Geometry: final body of the model. Coordinates: model frame, mm. Face numbers are marked on the shaded views. A direction names the side the tool comes from. Give positions to 0.01 mm unless a question says otherwise; leave off trailing zeros. Write each loop counter-clockwise with the first axis right and the second up, starting at its lowest first coordinate (ties: lowest second). Pieces come first, ordered by that corner, then holes.
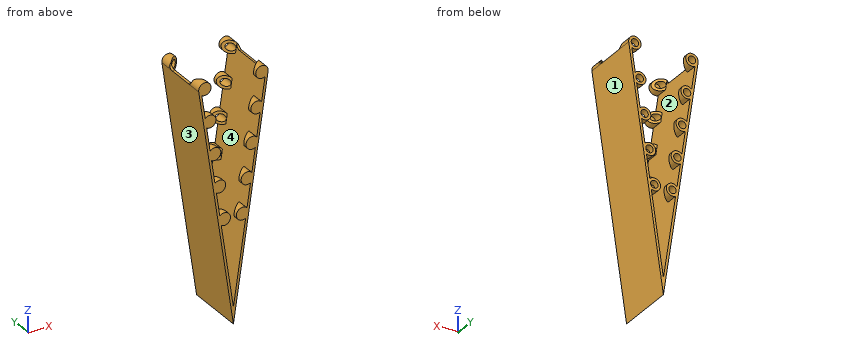
from build123d import *

# Parameters (mm, degrees)
BOSS_EXTRUDE1_DEPTH            = 25
SKETCH2_R                      = 2.6
SKETCH2_R_2                    = 1.55
BOSS_EXTRUDE3_DEPTH            = 5
CUT_EXTRUDE1_REACH             = 107.119
CUT_EXTRUDE1_DIRECTION_2_DEPTH = 106.119492302
CUT_EXTRUDE2_REACH             = 107.119
CUT_EXTRUDE2_DIRECTION_2_DEPTH = 106.119492302
FILLET1_R                      = 2
SKETCH6_R                      = 1.55
BOSS_EXTRUDE4_DEPTH            = 1


with BuildPart() as part:
    # Sketch1 → Boss-Extrude1 (new body)
    with BuildSketch(Plane(origin=(0, 0, 0), x_dir=(1, 0, 0), z_dir=(0, 1, 0))):
        Polygon((-13.5, 0), (0, 92.188031325), (13.5, 0), (14.489447114, 0.144894471), (0, 99.089605913), (-14.489447114, 0.144894471), align=None)
    extrude(amount=BOSS_EXTRUDE1_DEPTH)

    # Sketch2 → Boss-Extrude3 (add)
    # profile 1 of 10: a face of its own
    with BuildSketch(Plane(origin=(0, 0, 0), x_dir=(1, 0, 0), z_dir=(0, 1, 0))):
        with Locations((11.916884617, -0.231831154)):
            Circle(SKETCH2_R)
        with Locations(Location((11.916884617, -0.231831154, 0), (0, 0, 270))):
            Circle(SKETCH2_R_2, mode=Mode.SUBTRACT)
    # profile 2 of 10: a face of its own
    with BuildSketch(Plane(origin=(0, 0, 0), x_dir=(1, 0, 0), z_dir=(0, 1, 0))):
        with Locations((9.888362021, 13.620428448)):
            Circle(SKETCH2_R)
        with Locations(Location((9.888362021, 13.620428448, 0), (0, 0, 270))):
            Circle(SKETCH2_R_2, mode=Mode.SUBTRACT)
    # profile 3 of 10: a face of its own
    with BuildSketch(Plane(origin=(0, 0, 0), x_dir=(1, 0, 0), z_dir=(0, 1, 0))):
        with Locations((7.859839425, 27.47268805)):
            Circle(SKETCH2_R)
        with Locations(Location((7.859839425, 27.47268805, 0), (0, 0, 270))):
            Circle(SKETCH2_R_2, mode=Mode.SUBTRACT)
    # profile 4 of 10: a face of its own
    with BuildSketch(Plane(origin=(0, 0, 0), x_dir=(1, 0, 0), z_dir=(0, 1, 0))):
        with Locations((5.831316829, 41.324947652)):
            Circle(SKETCH2_R)
        with Locations(Location((5.831316829, 41.324947652, 0), (0, 0, 270))):
            Circle(SKETCH2_R_2, mode=Mode.SUBTRACT)
    # profile 5 of 10: a face of its own
    with BuildSketch(Plane(origin=(0, 0, 0), x_dir=(1, 0, 0), z_dir=(0, 1, 0))):
        with Locations((3.802794233, 55.177207254)):
            Circle(SKETCH2_R)
        with Locations(Location((3.802794233, 55.177207254, 0), (0, 0, 270))):
            Circle(SKETCH2_R_2, mode=Mode.SUBTRACT)
    # profile 6 of 10: a face of its own
    with BuildSketch(Plane(origin=(0, 0, 0), x_dir=(1, 0, 0), z_dir=(0, 1, 0))):
        with Locations((-11.916884617, -0.231831154)):
            Circle(SKETCH2_R)
        with Locations(Location((-11.916884617, -0.231831154, 0), (0, 0, 90))):
            Circle(SKETCH2_R_2, mode=Mode.SUBTRACT)
    # profile 7 of 10: a face of its own
    with BuildSketch(Plane(origin=(0, 0, 0), x_dir=(1, 0, 0), z_dir=(0, 1, 0))):
        with Locations((-9.888362021, 13.620428448)):
            Circle(SKETCH2_R)
        with Locations(Location((-9.888362021, 13.620428448, 0), (0, 0, 90))):
            Circle(SKETCH2_R_2, mode=Mode.SUBTRACT)
    # profile 8 of 10: a face of its own
    with BuildSketch(Plane(origin=(0, 0, 0), x_dir=(1, 0, 0), z_dir=(0, 1, 0))):
        with Locations((-7.859839425, 27.47268805)):
            Circle(SKETCH2_R)
        with Locations(Location((-7.859839425, 27.47268805, 0), (0, 0, 90))):
            Circle(SKETCH2_R_2, mode=Mode.SUBTRACT)
    # profile 9 of 10: a face of its own
    with BuildSketch(Plane(origin=(0, 0, 0), x_dir=(1, 0, 0), z_dir=(0, 1, 0))):
        with Locations((-5.831316829, 41.324947652)):
            Circle(SKETCH2_R)
        with Locations(Location((-5.831316829, 41.324947652, 0), (0, 0, 90))):
            Circle(SKETCH2_R_2, mode=Mode.SUBTRACT)
    # profile 10 of 10: a face of its own
    with BuildSketch(Plane(origin=(0, 0, 0), x_dir=(1, 0, 0), z_dir=(0, 1, 0))):
        with Locations((-3.802794233, 55.177207254)):
            Circle(SKETCH2_R)
        with Locations(Location((-3.802794233, 55.177207254, 0), (0, 0, 90))):
            Circle(SKETCH2_R_2, mode=Mode.SUBTRACT)
    boss_extrude3 = extrude(amount=BOSS_EXTRUDE3_DEPTH)

    # Cut-Extrude1: up to this face of the body (flat: up to its plane)
    cut_extrude1_end = Plane(part.part.faces().sort_by_distance((-6.65824674, 12.912249129, -46.7205751))[0])
    # Sketch4 → Cut-Extrude1 (cut, up to the picked face)
    with BuildSketch(Plane(origin=(0.283424505, 0, 1.935433121), x_dir=(0.9894471144188783, 0, -0.14489447114419254), z_dir=(0.14489447114419252, 0, 0.9894471144188782)), mode=Mode.PRIVATE) as cut_extrude1_sk1:
        Polygon((13.357536045, 5), (9.157536045, 5), (9.157536045, 1.475781549), align=None)
    cut_extrude1_tool1 = split(extrude(cut_extrude1_sk1.sketch, amount=-CUT_EXTRUDE1_REACH, mode=Mode.PRIVATE), bisect_by=cut_extrude1_end, keep=Keep.BOTH, mode=Mode.PRIVATE)
    cut_extrude1 = cut_extrude1_tool1.solids().sort_by(Axis((10.729548, 3.825261, 0.405705), (-0.14489447114419252, 0, -0.9894471144188782)))[0]
    add(cut_extrude1, mode=Mode.SUBTRACT)

    # Sketch4 → Cut-Extrude1 direction 2 (cut)
    with BuildSketch(Plane(origin=(0.283424505, 0, 1.935433121), x_dir=(0.9894471144188783, 0, -0.14489447114419254), z_dir=(0.14489447114419252, 0, 0.9894471144188782))):
        Polygon((13.357536045, 5), (9.157536045, 5), (9.157536045, 1.475781549), align=None)
    cut_extrude1_direction_2 = extrude(amount=CUT_EXTRUDE1_DIRECTION_2_DEPTH, mode=Mode.SUBTRACT)

    # Cut-Extrude2: up to this face of the body (flat: up to its plane)
    cut_extrude2_end = Plane(part.part.faces().sort_by_distance((6.65824674, 12.912249129, -46.7205751))[0])
    # Sketch5 → Cut-Extrude2 (cut, up to the picked face)
    with BuildSketch(Plane(origin=(-0.283424505, 0, 1.935433121), x_dir=(0.9894471144188784, 0, 0.14489447114419146), z_dir=(-0.14489447114419146, 0, 0.9894471144188784)), mode=Mode.PRIVATE) as cut_extrude2_sk1:
        Polygon((-9.157536045, 5), (-9.157536045, 1.475781549), (-13.357536045, 5), align=None)
    cut_extrude2_tool1 = split(extrude(cut_extrude2_sk1.sketch, amount=-CUT_EXTRUDE2_REACH, mode=Mode.PRIVATE), bisect_by=cut_extrude2_end, keep=Keep.BOTH, mode=Mode.PRIVATE)
    cut_extrude2 = cut_extrude2_tool1.solids().sort_by(Axis((-10.729548, 3.825261, 0.405705), (0.14489447114419146, 0, -0.9894471144188784)))[0]
    add(cut_extrude2, mode=Mode.SUBTRACT)

    # Sketch5 → Cut-Extrude2 direction 2 (cut)
    with BuildSketch(Plane(origin=(-0.283424505, 0, 1.935433121), x_dir=(0.9894471144188784, 0, 0.14489447114419146), z_dir=(-0.14489447114419146, 0, 0.9894471144188784))):
        Polygon((-9.157536045, 5), (-9.157536045, 1.475781549), (-13.357536045, 5), align=None)
    cut_extrude2_direction_2 = extrude(amount=CUT_EXTRUDE2_DIRECTION_2_DEPTH, mode=Mode.SUBTRACT)

    # Mirror2: Boss-Extrude3, Cut-Extrude1, Cut-Extrude1 direction 2, Cut-Extrude2, Cut-Extrude2 direction 2 across plane
    add(boss_extrude3.mirror(Plane.ZX.offset(12.5)))
    add(cut_extrude1.mirror(Plane.ZX.offset(12.5)), mode=Mode.SUBTRACT)
    add(cut_extrude1_direction_2.mirror(Plane.ZX.offset(12.5)), mode=Mode.SUBTRACT)
    add(cut_extrude2.mirror(Plane.ZX.offset(12.5)), mode=Mode.SUBTRACT)
    add(cut_extrude2_direction_2.mirror(Plane.ZX.offset(12.5)), mode=Mode.SUBTRACT)

    # Fillet1
    # the kernel refuses this fillet: 2 mm, written as the material it adds along each edge
    with BuildSketch(Plane(origin=(13.5, 5, 0), x_dir=(0, 1, 0), z_dir=(0.9894471144188783, 0, -0.1448944711441925))) as fillet1_piece_1_section:
        with BuildLine():
            CenterArc((FILLET1_R, FILLET1_R), FILLET1_R, 180, 90)
            Line((0, FILLET1_R), (0, 0))
            Line((0, 0), (FILLET1_R, 0))
        make_face()
    fillet1_piece_1 = extrude(amount=6, mode=Mode.PRIVATE)
    fillet1_piece_1 = fillet1_piece_1 & Plane(origin=(11.916884617, 5, 0.231831154), x_dir=(1, 0, 0), z_dir=(0, -1, 0)) * Cylinder(2.6, 20, mode=Mode.PRIVATE)
    add(fillet1_piece_1)
    with BuildSketch(Plane(origin=(13.5, 20, 0), x_dir=(0, -1, 0), z_dir=(0.9894471144188783, 0, -0.1448944711441925))) as fillet1_piece_2_section:
        with BuildLine():
            CenterArc((FILLET1_R, -FILLET1_R), FILLET1_R, 90, 90)
            Line((0, -FILLET1_R), (0, 0))
            Line((0, 0), (FILLET1_R, 0))
        make_face()
    fillet1_piece_2 = extrude(amount=6, mode=Mode.PRIVATE)
    fillet1_piece_2 = fillet1_piece_2 & Plane(origin=(11.916884617, 20, 0.231831154), x_dir=(1, 0, 0), z_dir=(0, 1, 0)) * Cylinder(2.6, 20, mode=Mode.PRIVATE)
    add(fillet1_piece_2)
    with BuildSketch(Plane(origin=(-19.436682687, 20, -0.869366827), x_dir=(0, -1, 0), z_dir=(0.9894471144188784, 0, 0.1448944711441914))) as fillet1_piece_3_section:
        with BuildLine():
            CenterArc((FILLET1_R, -FILLET1_R), FILLET1_R, 90, 90)
            Line((0, -FILLET1_R), (0, 0))
            Line((0, 0), (FILLET1_R, 0))
        make_face()
    fillet1_piece_3 = extrude(amount=6, mode=Mode.PRIVATE)
    fillet1_piece_3 = fillet1_piece_3 & Plane(origin=(-11.916884617, 20, 0.231831154), x_dir=(1, 0, 0), z_dir=(0, 1, 0)) * Cylinder(2.6, 21, mode=Mode.PRIVATE)
    add(fillet1_piece_3)
    with BuildSketch(Plane(origin=(-19.436682687, 5, -0.869366827), x_dir=(-0.1448944711441914, 0, 0.9894471144188784), z_dir=(0.9894471144188784, 0, 0.1448944711441914))) as fillet1_piece_4_section:
        with BuildLine():
            CenterArc((FILLET1_R, -FILLET1_R), FILLET1_R, 90, 90)
            Line((0, -FILLET1_R), (0, 0))
            Line((0, 0), (FILLET1_R, 0))
        make_face()
    fillet1_piece_4 = extrude(amount=6, mode=Mode.PRIVATE)
    fillet1_piece_4 = fillet1_piece_4 & Plane(origin=(-11.916884617, 5, 0.231831154), x_dir=(1, 0, 0), z_dir=(0, -1, 0)) * Cylinder(2.6, 21, mode=Mode.PRIVATE)
    add(fillet1_piece_4)

    # Sketch6 → Boss-Extrude4 (add)
    with BuildSketch(Plane.XZ):
        with Locations(Location((3.802794233, -55.177207254, 0), (0, 0, 270))):
            Circle(SKETCH6_R)
        with Locations(Location((-3.802794233, -55.177207254, 0), (0, 0, 270))):
            Circle(SKETCH6_R)
        with Locations(Location((-5.831316829, -41.324947652, 0), (0, 0, 270))):
            Circle(SKETCH6_R)
        with Locations(Location((5.831316829, -41.324947652, 0), (0, 0, 270))):
            Circle(SKETCH6_R)
        with Locations(Location((7.859839425, -27.47268805, 0), (0, 0, 270))):
            Circle(SKETCH6_R)
        with Locations(Location((-7.859839425, -27.47268805, 0), (0, 0, 270))):
            Circle(SKETCH6_R)
        with Locations(Location((-9.888362021, -13.620428448, 0), (0, 0, 270))):
            Circle(SKETCH6_R)
        with Locations(Location((9.888362021, -13.620428448, 0), (0, 0, 270))):
            Circle(SKETCH6_R)
        with Locations(Location((11.916884617, 0.231831154, 0), (0, 0, 270))):
            Circle(SKETCH6_R)
        with Locations(Location((-11.916884617, 0.231831154, 0), (0, 0, 270))):
            Circle(SKETCH6_R)
    extrude(amount=-BOSS_EXTRUDE4_DEPTH)


solid = part.part
Q1. Access query for the marked faces 3 and 4. Directions: +Z, -Z, +X, -X, +Y, -Y. A direction counts if a zero-diameter tool reaches every point of the face in a straight line with its end or side. Return the directions, or none.
Filled sheet:
face 3: -Z, -X, +Y, -Y
face 4: none
Q2. Section B-B on y = 15.75. Output: boundary loops of the cut face in (x, z), plus the area to 3 significant figures.
Filled sheet:
outline: (-14.49, -0.14) - (0, -99.09) - (14.49, -0.14) - (13.5, 0) - (0, -92.19) - (-13.5, 0) - close
area: 193 mm2
Q3. Pull-direction query (Y, two-part tool) for the marked faces 1 and 2; classes: released by +Y, released by -Y, zero draft, split by the parting line, or undercut.
Filled sheet:
face 1: zero draft
face 2: undercut
Q4. Ray query, line 1 along X through (y, z) = (1.25, -55.5); line 2 along X through (y, z) = (10, -61); line 3 along X through (y, z) = (6.5, -75). Return the intervals inside material, ascending.
Filled sheet:
line 1: x = -6.38 to -5.32, -2.29 to -1.22, 1.22 to 2.29, 5.32 to 6.38
line 2: x = -5.58 to -4.57, 4.57 to 5.58
line 3: x = -3.53 to -2.52, 2.52 to 3.53
Q5. Section A-A on z = -60. Output: boundary loops of the cut face in (x, y).
Filled sheet:
outline: (-5.72, 0) - (-4.71, 0) - (-4.71, 25) - (-5.72, 25) - close; (4.71, 0) - (5.72, 0) - (5.72, 25) - (4.71, 25) - close
Q6. Pin query (flat end, axial travel): P1, Ø0.9, axis at x = 8.5, z = -28, coming from the +Y side; P2, Ø4, axis at y = 3, z = -75, coming from the -X side; P3, Ø1.5, axis at y = 13.5, z = -73, coming from the +X side. Return the tip coordinate at first contact, or that it passes through.
Filled sheet:
P1: stops at y = 1
P2: stops at x = -3.82
P3: stops at x = 3.93
